from build123d import *

# Parameters (mm, degrees)
BOSS_EXTRUDE1_DEPTH = 30
CHAMFER1_SIZE       = 0.5
CHAMFER2_SIZE       = 0.5
CHAMFER3_SIZE       = 0.5


with BuildPart() as part:
    # Sketch1 → Boss-Extrude1 (new body)
    with BuildSketch(Plane(origin=(0, 0, 0), x_dir=(0, 0, -1), z_dir=(1, 0, 0))):
        Polygon((0, 2.309401077), (-2, 1.154700538), (-2, -1.154700538), (0, -2.309401077), (2, -1.154700538), (2, 1.154700538), align=None)
    extrude(amount=BOSS_EXTRUDE1_DEPTH)

    # Sketch4 → Revolve4 (revolve)
    with BuildSketch(Plane.XY):
        Polygon((0, 0), (-5, 0), (-5, 5), (-3.25, 5), (-1.25, 2.309401077), (0, 2.309401077), align=None)
    revolve(axis=Axis((0, 0, 0), (-1, 0, 0)))

    # Chamfer1
    # the kernel refuses this chamfer: 0.5 mm, written as the material it adds along each edge
    with BuildSketch(Plane(origin=(0, -2.952321824, 1.113571399), x_dir=(0.9996219169112968, 0.02381212764409037, 0.013747938305293311), z_dir=(0, 0.5000000000000001, -0.8660254037844386))) as chamfer1_piece_1_section:
        Polygon((CHAMFER1_SIZE * 0.999621916911, CHAMFER1_SIZE * 0.0274958766106), (-CHAMFER1_SIZE * 0.0274958766106, CHAMFER1_SIZE * 0.999621916911), (0, 0), align=None)
    chamfer1_piece_1 = extrude(amount=4.881084065, mode=Mode.PRIVATE)
    chamfer1_piece_1 = split(chamfer1_piece_1, bisect_by=Plane(origin=(0.199770768, -1.81784162, -2), z_dir=(0, 0, 1)), keep=Keep.TOP, mode=Mode.PRIVATE)
    chamfer1_piece_1 = split(chamfer1_piece_1, bisect_by=Plane(origin=(0.199770768, -2.640971617, -0.574297023), z_dir=(0, 0.8660254037844387, -0.49999999999999983)), keep=Keep.TOP, mode=Mode.PRIVATE)
    chamfer1_piece_1 = chamfer1_piece_1 & Plane(origin=(0.199770768, 0, 0), x_dir=(0, 1, 0), z_dir=(1, 0, 0)) * Cylinder(2.309401077, 12, mode=Mode.PRIVATE)
    add(chamfer1_piece_1)
    with BuildSketch(Plane(origin=(0, 2.952321824, -1.113571399), x_dir=(0.9996219169112968, -0.023812127644089905, -0.013747938305293039), z_dir=(0, -0.5000000000000001, 0.8660254037844387))) as chamfer1_piece_2_section:
        Polygon((CHAMFER1_SIZE * 0.999621916911, CHAMFER1_SIZE * 0.0274958766106), (-CHAMFER1_SIZE * 0.0274958766106, CHAMFER1_SIZE * 0.999621916911), (0, 0), align=None)
    chamfer1_piece_2 = extrude(amount=4.881084065, mode=Mode.PRIVATE)
    chamfer1_piece_2 = split(chamfer1_piece_2, bisect_by=Plane(origin=(0.19977077, 2.640971618, 0.574297023), z_dir=(0, -0.8660254037844388, 0.49999999999999983)), keep=Keep.TOP, mode=Mode.PRIVATE)
    chamfer1_piece_2 = split(chamfer1_piece_2, bisect_by=Plane(origin=(0.19977077, 1.817841619, 2), z_dir=(0, 0, -1)), keep=Keep.TOP, mode=Mode.PRIVATE)
    chamfer1_piece_2 = chamfer1_piece_2 & Plane(origin=(0.19977077, 0, 0), x_dir=(0, 1, 0), z_dir=(1, 0, 0)) * Cylinder(2.309401077, 12, mode=Mode.PRIVATE)
    add(chamfer1_piece_2)

    # Chamfer2
    # the kernel refuses this chamfer: 0.5 mm, written as the material it adds along each edge
    with BuildSketch(Plane(origin=(0, -2.440542032, -2), x_dir=(0.9996219169112968, 0, 0.027495876610586494), z_dir=(0, 1, 0))) as chamfer2_piece_1_section:
        Polygon((CHAMFER2_SIZE * 0.999621916911, CHAMFER2_SIZE * 0.0274958766106), (-CHAMFER2_SIZE * 0.0274958766106, CHAMFER2_SIZE * 0.999621916911), (0, 0), align=None)
    chamfer2_piece_1 = extrude(amount=4.881084065, mode=Mode.PRIVATE)
    chamfer2_piece_1 = chamfer2_piece_1 & Plane(origin=(0.352657497, 0, 0), x_dir=(0, 1, 0), z_dir=(1, 0, 0)) * Cylinder(2.309401077, 12, mode=Mode.PRIVATE)
    chamfer2_piece_1 = split(chamfer2_piece_1, bisect_by=Plane(origin=(0.352657497, 0.578909499, -2.997299335), z_dir=(0, -0.8660254037844388, 0.49999999999999983)), keep=Keep.TOP, mode=Mode.PRIVATE)
    add(chamfer2_piece_1)
    with BuildSketch(Plane(origin=(0, 2.440542032, 2), x_dir=(0.9996219169112968, 0, -0.027495876610586494), z_dir=(0, -1, 0))) as chamfer2_piece_2_section:
        Polygon((CHAMFER2_SIZE * 0.999621916911, CHAMFER2_SIZE * 0.0274958766106), (-CHAMFER2_SIZE * 0.0274958766106, CHAMFER2_SIZE * 0.999621916911), (0, 0), align=None)
    chamfer2_piece_2 = extrude(amount=4.881084065, mode=Mode.PRIVATE)
    chamfer2_piece_2 = chamfer2_piece_2 & Plane(origin=(0.352657497, 0, 0), x_dir=(0, 1, 0), z_dir=(1, 0, 0)) * Cylinder(2.309401077, 12, mode=Mode.PRIVATE)
    chamfer2_piece_2 = split(chamfer2_piece_2, bisect_by=Plane(origin=(0.352657497, -0.578909499, 2.997299335), z_dir=(0, 0.8660254037844387, -0.49999999999999983)), keep=Keep.TOP, mode=Mode.PRIVATE)
    add(chamfer2_piece_2)

    # Chamfer3
    # the kernel refuses this chamfer: 0.5 mm, written as the material it adds along each edge
    with BuildSketch(Plane(origin=(0, 0.511779791, -3.113571399), x_dir=(-0.027495876610586466, 0.8656979742248804, -0.49981095845564816), z_dir=(0, 0.49999999999999983, 0.8660254037844388))) as chamfer3_piece_1_section:
        Polygon((CHAMFER3_SIZE * 0.999621916911, -CHAMFER3_SIZE * 0.0274958766106), (-CHAMFER3_SIZE * 0.0274958766106, -CHAMFER3_SIZE * 0.999621916911), (0, 0), align=None)
    chamfer3_piece_1 = extrude(amount=4.881084065, mode=Mode.PRIVATE)
    chamfer3_piece_1 = chamfer3_piece_1 & Plane(origin=(0.352657492, 0, 0), x_dir=(0, 1, 0), z_dir=(1, 0, 0)) * Cylinder(2.309401077, 12, mode=Mode.PRIVATE)
    add(chamfer3_piece_1)
    with BuildSketch(Plane(origin=(0, -0.511779791, 3.113571399), x_dir=(0.9996219169112968, 0.023812127644090055, -0.013747938305293115), z_dir=(0, -0.4999999999999999, -0.8660254037844388))) as chamfer3_piece_2_section:
        Polygon((CHAMFER3_SIZE * 0.999621916911, CHAMFER3_SIZE * 0.0274958766106), (-CHAMFER3_SIZE * 0.0274958766106, CHAMFER3_SIZE * 0.999621916911), (0, 0), align=None)
    chamfer3_piece_2 = extrude(amount=4.881084065, mode=Mode.PRIVATE)
    chamfer3_piece_2 = chamfer3_piece_2 & Plane(origin=(0.352657501, 0, 0), x_dir=(0, 1, 0), z_dir=(1, 0, 0)) * Cylinder(2.309401077, 12, mode=Mode.PRIVATE)
    add(chamfer3_piece_2)


solid = part.part
Can you work these out from the model? Positions are in its coordinate system, mm. A direction names the side the tool comes from. Give positions to 0.01 mm unless a question says otherwise; leave off trailing zeros. Write each loop counter-clockwise with the first axis right and the second up, starting at its lowest first coordinate (ties: lowest second). Pieces come first, ordered by that corner, then holes. Notation, with made-up numbers: M 0.5,18 L 41.5,18 A21 cw 41.5,27 Z; hole C -16,1.5 d5. An arc over 180 degrees is marked long. Answer in a Markdown table with one row per item. Add a question column.
Item 1: Please list where these lines run through material, in increasing order: L1, parallel to Z at x = 27, y = -0.5; L2, parallel to X at y = -2.5, z = -2.5; L3, parallel to Y at x = -2, z = 0.25.
Item 2: Imagine slicing it at A-A, the plane y = 0. Write out the boundary of the cut face in (x, z), plus the area to 3 significant figures.
Item 3: On a 3-axis mill with a long thin cutter (end or side, diameter ignored), from which of +Z, -Z, +X, -X, +Y, -Y can I reach the whole of each face in a straight line? I mean faces 1 (the flat face through (15.04, -1.74, -0.99)), 2 (the flat face through (15.043, -1.724, 1.014)), 3 (the flat face through (15.04, 1.74, 0.99)), 4 (the flat face through (15.043, 1.724, -1.014)), 5 (the flat face through (15, 0, -2)). Say none if no direction works.
Item 4: For pin 1 Ø1.5 at (x, y) = (23, -4) entering from +Z; pin 2 Ø2.5 at (x, y) = (9, 0) entering from +Z; pin 3 Ø0.7 at (x, y) = (11, 0.5) entering from -Z; pin 4 Ø2 at (y, z) = (2, 4) entering from +X, each with a flat end and sliding along its axis, tell me the tip position at first contact or that it passes through.
Item 5: Imagine slicing it at B-B, the plane x = 23. Write out the boundary of the cut face in (y, z), plus the area to 3 significant figures.
Evaluation:
| question | item | result |
|---|---|---|
| 1 | L1 | z = -2 to 2 |
| 1 | L2 | x = -5 to -2.16 |
| 1 | L3 | y = -3.31 to 3.31 |
| 2 | outline | M -5,-5 L -3.25,-5 L -1.25,-2.31 L 0.19,-2.31 L 0.5,-2 L 30,-2 L 30,2 L 0.5,2 L 0.19,2.31 L -1.25,2.31 L -3.25,5 L -5,5 Z |
| 2 | area | 158 mm² |
| 3 | face 1 | -Z, +X, -Y |
| 3 | face 2 | +Z, +X, -Y |
| 3 | face 3 | +Z, +X, +Y |
| 3 | face 4 | -Z, +X, +Y |
| 3 | face 5 | -Z, +X, +Y, -Y |
| 4 | pin 1 | passes through |
| 4 | pin 2 | stops at z = 2 |
| 4 | pin 3 | stops at z = -2 |
| 4 | pin 4 | stops at x = -2.11 |
| 5 | outline | M -2.31,0 L -1.15,-2 L 1.15,-2 L 2.31,0 L 1.15,2 L -1.15,2 Z |
| 5 | area | 13.9 mm² |
